Study the drawing (mm; zero at the part's minimum x, y, z) and answer. A direction names the side the tool comes from. Coordinates: 2 decimals unless noted, no trailing zeros. Loops run counter-clockwise (first coordinate to the right, second up) from the corner with the lowest first, then second, coordinate; pieces in that order, holes last. Notation, with made-up numbers: (-16.5, -7) - (15.5, -7) arc R19 ccw to (15.5, 0) - close; hole circle Ø6 at (89, 63). An arc over 180 degrees is marked (long way). Write each question's results on one line, items separated by ' | '. Start each with the question number.
(1) Consider line 1 (X direction, y = 3.55, z = 5.2); line 2 (Y direction, x = 7.25, z = 5.3). Determine where each line is inside the solid, lowest interval first. Write a range as from..to.
(2) Find section B-B on z = 3.4. Determine the outline of the cut face in (x, y).
(3) Find section A-A on y = 5.65. Determine the outline of the cut face in (x, z), then the cut area to 3 significant figures.
(4) Given pin 1 Ø3 at (x, z) = (7.5, 1.5) entering from +Y, flat-ended and moving along its own axis, determine where the tip first touches the part or whether it passes through.
(5) Find section C-C on x = 4.75. Determine the outline of the cut face in (y, z), then the cut area to 3 significant figures.
(6) Determine the mould class of the marked faces 3, 4 and 5 for opening direction X: released by +X, released by -X, zero draft, split by the parting line, or undercut.
(7) For the marked faces 1 and 2, determine the directions among +Z, -Z, +X, -X, +Y, -Y from which every point of the face is accessible in a straight line to the end or side of a thin tool.
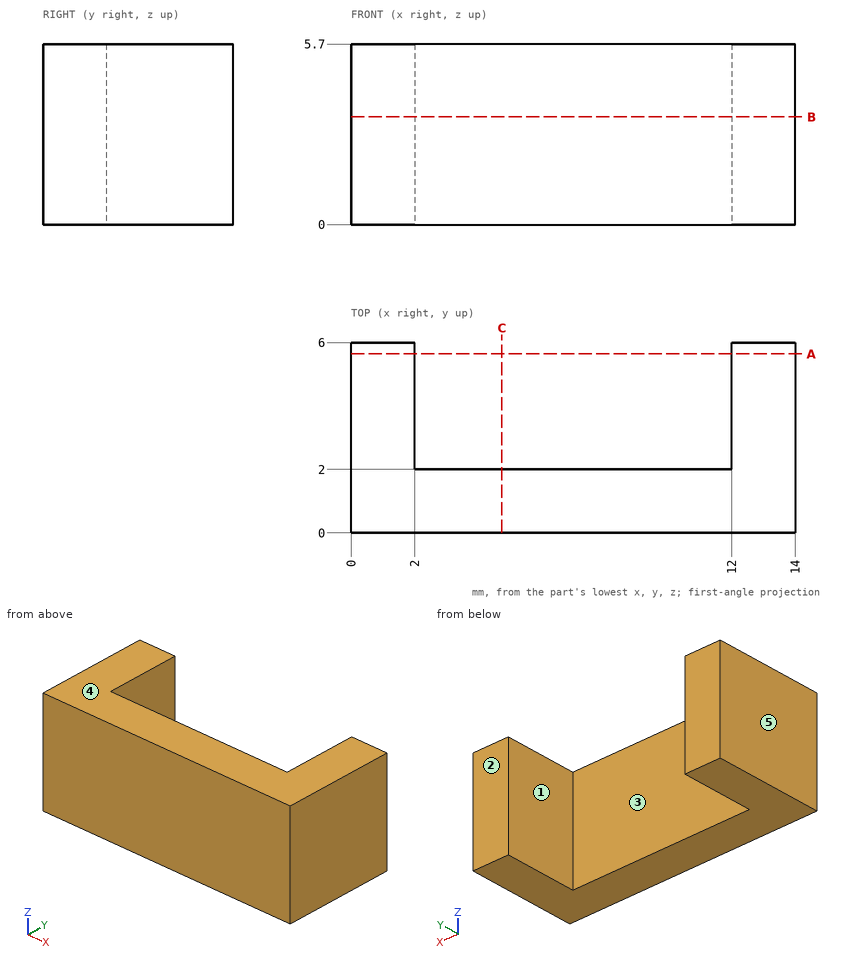
Values:
1) line 1: x = 0..2, 12..14 | line 2: y = 0..2
2) outline: (0, 0) - (14, 0) - (14, 6) - (12, 6) - (12, 2) - (2, 2) - (2, 6) - (0, 6) - close
3) outline: (0, 0) - (2, 0) - (2, 5.7) - (0, 5.7) - close; (12, 0) - (14, 0) - (14, 5.7) - (12, 5.7) - close | area: 22.8 mm²
4) pin 1: stops at y = 2
5) outline: (0, 0) - (2, 0) - (2, 5.7) - (0, 5.7) - close | area: 11.4 mm²
6) face 3: undercut | face 4: zero draft | face 5: released by -X
7) face 1: +Z, -Z, +Y | face 2: +Z, -Z, +X, -X, +Y
